The listing builds one solid part. Answer for the finished solid, in the listing's coordinates (mm). Coordinates: 2 decimals unless noted, no trailing zeros. Order: outer loops, then holes, each group sorted by start corner. A loop starts at its lowest first (then second) coordinate and runs counter-clockwise, first axis right, second up. Notation, with made-up numbers: (-13.5, -36.75) - (29.5, -36.75) arc R11 ccw to (29.5, -29.75) - close; hole circle Ø1 at (70, 20). An arc over 180 degrees is marked (long way). Use a Markdown table: item, result. Add a question column.
Item 1: The part is cut by section A-A, the plane z = 21. Give the vertices of the cut face in (x, y).
Item 2: The part is cut by section B-B, the plane x = 1. Give the vertices of the cut face in (y, z).
Item 3: The part is cut by section C-C, the plane y = -1.55. State how many separate pieces and enclosed holes the cut face has, then the cut area to 3 significant figures.
Item 4: Find the intervals of material crossed by line 1 along X through (y, z) = (-2, -41); line 2 along X through (y, z) = (1.7, 22); line 3 along X through (y, z) = (-1.8, 20.5), in increasing order.
Item 5: A flat-ended cylindrical pin translates along its axis: P1, Ø1, axis at x = -29, z = 9, coming from the -Y side. Find the tip coordinate at first contact, or state that the pin passes through.
Item 6: The part is cut by section D-D, the plane z = -29. Give the vertices of the cut face in (x, y).
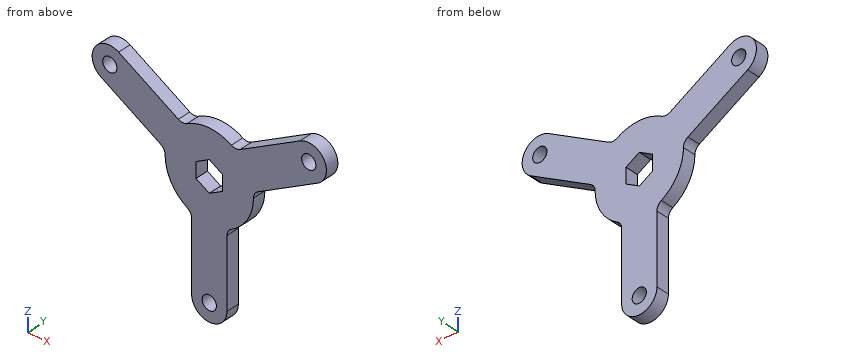
from build123d import *

# Parameters (mm, degrees)
SKETCH1_R                = 15.875
BOSS_EXTRUDE1_DEPTH      = 2.3495
SKETCH2_R                = 2.5527
BOSS_EXTRUDE2_DEPTH      = 4.699
FILLET1_R                = 3.175
CIRPATTERN1_COUNT        = 3
FILLET1_OF_CIRPATTERN1_R = 3.175


with BuildPart() as part:
    # Sketch1 → Boss-Extrude1 (new, symmetric)
    with BuildSketch(Plane(origin=(0, 0, 0), x_dir=(1, 0, 0), z_dir=(0, 1, 0))):
        with Locations(Location((0, 0, 0), (0, 0, 270))):
            Circle(SKETCH1_R)
        Polygon((0, 5.499261314), (-4.7625, 2.749630657), (-4.7625, -2.749630657), (0, -5.499261314), (4.7625, -2.749630657), (4.7625, 2.749630657), align=None, mode=Mode.SUBTRACT)
    extrude(amount=BOSS_EXTRUDE1_DEPTH, both=True)

    # Sketch2 → Boss-Extrude2 (add)
    with BuildSketch(Plane(origin=(0, 2.3495, 0), x_dir=(1, 0, 0), z_dir=(0, 1, 0))):
        with BuildLine():
            Line((-6.35, 41.275), (-6.35, 14.549677831))
            ThreePointArc((-6.35, 14.549677831), (0, 15.875), (6.35, 14.549677831))
            Line((6.35, 14.549677831), (6.35, 41.275))
            ThreePointArc((6.35, 41.275), (0, 47.625), (-6.35, 41.275))
        make_face()
        with Locations(Location((0, 41.275, 0), (0, 0, 270))):
            Circle(SKETCH2_R, mode=Mode.SUBTRACT)
    boss_extrude2 = extrude(amount=-BOSS_EXTRUDE2_DEPTH)

    # Fillet1
    fillet1_edges = [part.edges().sort_by_distance(p)[0] for p in [
        (-6.35, 0, -14.549677831),
        (6.35, 0, -14.549677831),
    ]]
    fillet(fillet1_edges, radius=FILLET1_R)

    # CirPattern1: Boss-Extrude2 ×3 about axis
    cirpattern1_axis = Axis((0, 0, 0), (0, 1, 0))
    for i in range(1, CIRPATTERN1_COUNT):
        add(boss_extrude2.rotate(cirpattern1_axis, i * 360 / CIRPATTERN1_COUNT))

    # Fillet1 of CirPattern1
    fillet1_of_cirpattern1_edges = [part.edges().sort_by_distance(p)[0] for p in [
        (-9.425390619, 0, 12.77410023),
        (-15.775390619, 0, 1.775577602),
        (15.775390619, 0, 1.775577602),
        (9.425390619, 0, 12.77410023),
    ]]
    fillet(fillet1_of_cirpattern1_edges, radius=FILLET1_OF_CIRPATTERN1_R)


solid = part.part
Solution:
| question | item | result |
|---|---|---|
| 1 | outline | (-42.08, -2.35) - (-38.27, -2.35) - (-38.27, 2.35) - (-42.08, 2.35) - close; (-33.22, -2.35) - (-23.67, -2.35) - (-23.67, 2.35) - (-33.22, 2.35) - close; (23.67, -2.35) - (33.22, -2.35) - (33.22, 2.35) - (23.67, 2.35) - close; (38.27, -2.35) - (42.08, -2.35) - (42.08, 2.35) - (38.27, 2.35) - close |
| 2 | outline | (-2.35, -47.55) - (2.35, -47.55) - (2.35, -43.62) - (-2.35, -43.62) - close; (-2.35, -38.93) - (2.35, -38.93) - (2.35, -4.92) - (-2.35, -4.92) - close; (-2.35, 4.92) - (2.35, 4.92) - (2.35, 15.84) - (-2.35, 15.84) - close |
| 3 | separate pieces | 1 |
| 3 | enclosed holes | 4 |
| 3 | area | 1,830 mm2 |
| 4 | line 1 | x = -6.35 to -2.54, 2.54 to 6.35 |
| 4 | line 2 | x = -41.95 to -37.9, -33.59 to -25.41, 25.41 to 33.59, 37.9 to 41.95 |
| 4 | line 3 | x = -42.09 to -38.29, -33.2 to -22.81, 22.81 to 33.2, 38.29 to 42.09 |
| 5 | P1 | stops at y = -2.35 |
| 6 | outline | (-6.35, -2.35) - (6.35, -2.35) - (6.35, 2.35) - (-6.35, 2.35) - close |
